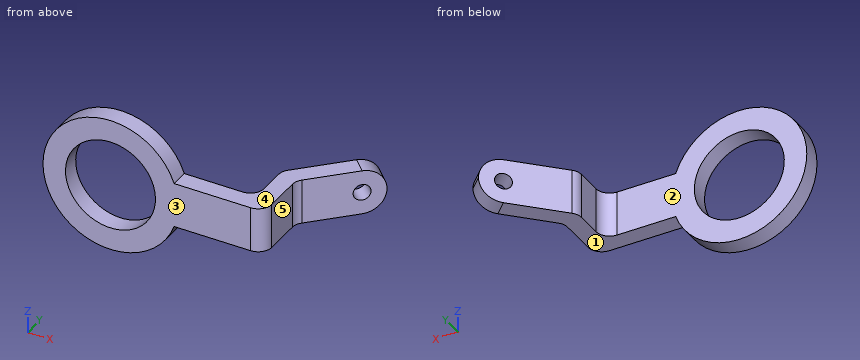
```python
from build123d import *

# Parameters (mm, degrees)
SKETCH2_R            = 10
BOSS_EXTRUDE1_DEPTH  = 4
BOSS_EXTRUDE2_DEPTH  = 10
FILLET1_R            = 5
M3_CLEARANCE_HOLE1_D = 3.6
FILLET2_R            = 3


with BuildPart() as part:
    # Sketch2 → Boss-Extrude1 (new body)
    with BuildSketch(Plane(origin=(0, 0, 0), x_dir=(1, 0, 0), z_dir=(0, 1, 0))):
        with BuildLine():
            Line((34.142135624, 5), (34.142135624, -5))
            Line((34.142135624, -5), (14.142135624, -5))
            ThreePointArc((14.142135624, -5), (-15, 0), (14.142135624, 5))
            Line((14.142135624, 5), (34.142135624, 5))
        make_face()
        with Locations(Location((0, 0, 0), (0, 0, 270))):
            Circle(SKETCH2_R, mode=Mode.SUBTRACT)
    extrude(amount=BOSS_EXTRUDE1_DEPTH)

    # Sketch3 → Boss-Extrude2 (add)
    with BuildSketch(Plane.XY.offset(5)):
        Polygon((34.142135624, 4), (34.142135624, 12.343145751), (47.112698372, 25.313708499), (44.284271247, 28.142135624), (30.142135624, 14), (30.142135624, 4), align=None)
    extrude(amount=-BOSS_EXTRUDE2_DEPTH)

    # Fillet1
    fillet1_edges = [part.edges().sort_by_distance(p)[0] for p in [
        (45.69848481, 26.727922061, 5),
        (45.69848481, 26.727922061, -5),
    ]]
    fillet(fillet1_edges, radius=FILLET1_R - 0.0001)  # a hair under: the kernel refuses the full size

    # M3 Clearance Hole1 (through all)
    with Locations(Plane(origin=(8.071067812, -8.071067812, 0), x_dir=(0.7071067811865486, 0.7071067811865465, 0), z_dir=(-0.7071067811865465, 0.7071067811865486, 0))):
        with Locations((46.213203436, 0)):
            Hole(M3_CLEARANCE_HOLE1_D / 2)

    # Fillet2
    fillet2_edges = [part.edges().sort_by_distance(p)[0] for p in [
        (30.142135624, 4, 0),
        (30.142135624, 14, 0),
        (34.142135624, 12.343145751, 0),
        (34.142135624, 0, 0),
    ]]
    fillet(fillet2_edges, radius=FILLET2_R)


solid = part.part
```
Geometry: final body of the model. Coordinates: model frame, mm. Face numbers are marked on the shaded views. A direction names the side the tool comes from. Round coordinates to 2 decimals unless told otherwise and drop trailing zeros. Order: outer loops, then holes, each group sorted by start corner. A loop starts at its lowest first (then second) coordinate and runs counter-clockwise, first axis right, second up. Notation, with made-up numbers: M 5,49.5 L 40,49.5 A27 cw 40,65.5 Z; hole C 12,37 d4. An arc over 180 degrees is marked long. One line per item, written item: value.
(1) Pin query (flat end, axial travel): P1, Ø2.5, axis at y = 8, z = 0, coming from the +X side; P2, Ø6, axis at x = -3.5, z = -4.5, coming from the -Y side; P3, Ø2, axis at y = 12.5, z = 4, coming from the +X side; P4, Ø6.5, axis at y = 8.5, z = 1, coming from the -X side. Return the tip coordinate at first contact, or that it passes through.
Result sheet:
P1: x = 34.14
P2: through
P3: x = 35.3
P4: x = 29.58
(2) Cut plane D-D (z = 11.5). Return the cut outline in (x, y).
Result sheet:
outline: M -9.63,0 L 9.63,0 L 9.63,4 L -9.63,4 Z
(3) Cut plane A-A (x = 0). Return the cut outline in (y, z).
Result sheet:
outline: M 0,-15 L 4,-15 L 4,-10 L 0,-10 Z; M 0,10 L 4,10 L 4,15 L 0,15 Z
(4) Reachability of the marked faces 1, 2, 3, 4 and 5 from +Z, -Z, +X, -X, +Y, -Y: full face, straight path, thin tool, end or side. Return the list, or none.
Result sheet:
face 1: -Z, +X, +Y, -Y
face 2: +Z, -Z, -X, +Y
face 3: +Z, -Z, +X, -X, -Y
face 4: +Z, +X, +Y, -Y
face 5: +Z, -Z, +X, -Y
(5) Cut plane B-B (z = -3.5). Return the cut outline in (x, y).
Result sheet:
outline: M -14.59,0 L -9.37,0 L -9.37,4 L -14.59,4 Z; M 9.37,0 L 31.14,0 A3 ccw 34.14,3 L 34.14,11.1 A3 cw 35.02,13.22 L 46.1,24.3 L 43.27,27.13 L 31.02,14.88 A3 ccw 30.14,12.76 L 30.14,7 A3 cw 27.14,4 L 9.37,4 Z
(6) Line query: probe 1 along X at (y, z) = (2.9, 0); probe 2 along Z at (x, y) = (17, 2.5); probe 3 along Y at (x, z) = (-3, 11.5). Output: solid intervals per line, ascending. Write a range as [from, to].
Result sheet:
probe 1: [-15, -10], [10, 34.14]
probe 2: [-5, 5]
probe 3: [0, 4]
(7) Cut plane C-C (y = 8.75). Return the cut outline in (x, z), and give its area (3 significant figures).
Result sheet:
outline: M 30.14,-5 L 34.14,-5 L 34.14,5 L 30.14,5 Z
area: 40.0 mm2
